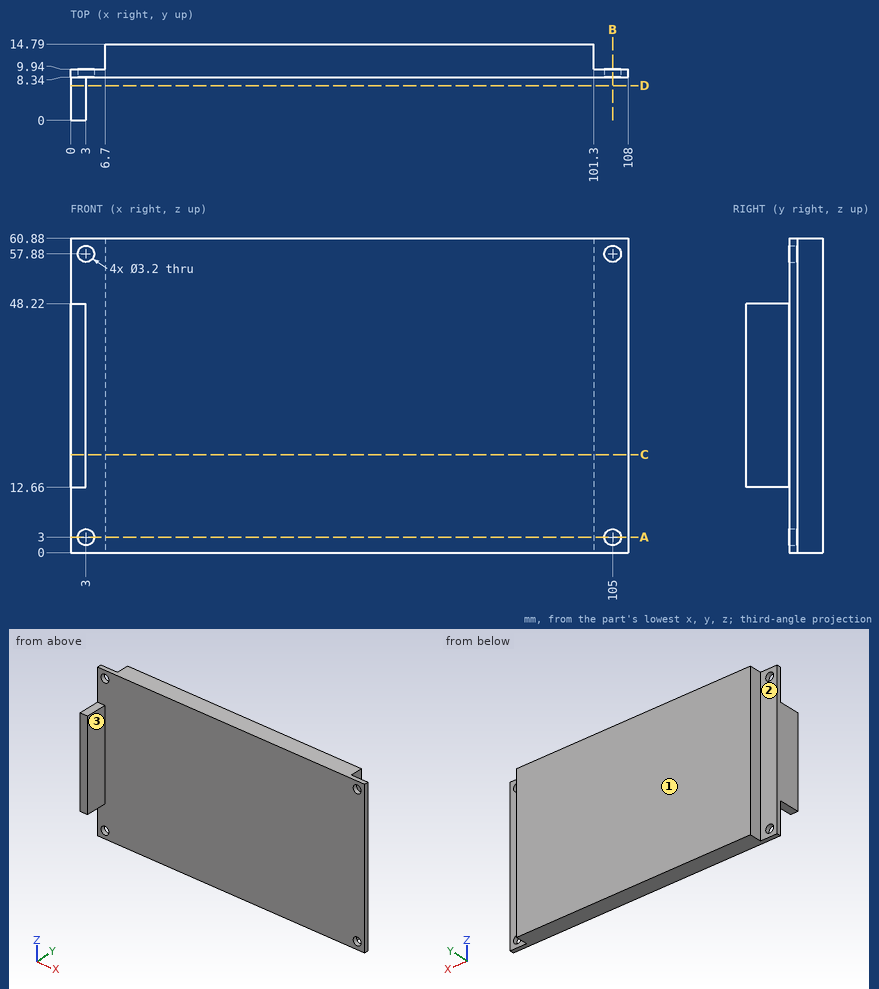
The figure shows three views and two pictorial views of one solid part (mm, origin at its lowest corner). Answer the questions. A direction names the side the tool comes from. Round coordinates to 2 decimals unless told otherwise and drop trailing zeros. Write each loop counter-clockwise with the first axis right and the second up, starting at its lowest first coordinate (ties: lowest second). Pieces come first, ordered by that corner, then holes. Notation, with made-up numbers: (-31, 5.5) -> (9, 5.5) arc R18 cw to (9, 13.5) -> close; hole circle Ø10 at (3, 42.5). An arc over 180 degrees is marked (long way). Write each question's results on one line, items separated by ' | '.
Q1. Section B-B, the plane x = 105 is taken. Write down the section's boundary in (y, z).
Data:
outline: (8.34, 0) -> (9.94, 0) -> (9.94, 1.4) -> (8.34, 1.4) -> close; (8.34, 4.6) -> (9.94, 4.6) -> (9.94, 56.28) -> (8.34, 56.28) -> close; (8.34, 59.48) -> (9.94, 59.48) -> (9.94, 60.88) -> (8.34, 60.88) -> close
Q2. Section C-C, the plane z = 19 is taken. Write down the section's boundary in (x, y).
Data:
outline: (0, 0) -> (3, 0) -> (3, 8.34) -> (108, 8.34) -> (108, 9.94) -> (101.3, 9.94) -> (101.3, 14.79) -> (6.7, 14.79) -> (6.7, 9.94) -> (0, 9.94) -> close
Q3. Flat-ended cylindrical pins translate along their axes: P1, Ø18.5, axis at x = 42, z = 28, coming from the -Y side; P2, Ø0.9, axis at x = 1.5, y = 2.5, coming from the -Z side; P3, Ø5.5, axis at y = 12, z = 19.5, coming from the -X side; P4, Ø3.5, axis at x = 104.5, z = 37, coming from the +Y side. Find the tip coordinate at first contact, or state that the pin passes through.
Data:
P1: y = 8.34 | P2: z = 12.66 | P3: x = 0 | P4: y = 9.94
Q4. Which of the six approach directions +Z, -Z, +X, -X, +Y, -Y give full straight-line access (tool end or side, diameter ignored) to the marked faces 1, 2 and 3?
Data:
face 1: +Z, -Z, +X, -X, +Y | face 2: +Z, -Z, -X, +Y | face 3: +Z, -Z, +X, -Y
Q5. Straight lines are drawn through the part: line 1 along X through (y, z) = (9.05, 3); line 2 along Z through (x, y) = (105, 8.75); line 3 along X through (y, z) = (5.25, 16.5). For each, find the intervals that lie inside material, in ascending order. Write a range as [from, to].
Data:
line 1: [0, 1.4], [4.6, 103.4], [106.6, 108] | line 2: [0, 1.4], [4.6, 56.28], [59.48, 60.88] | line 3: [0, 3]
Q6. Section A-A, the plane z = 3 is taken. Write down the section's boundary in (x, y).
Data:
outline: (0, 8.34) -> (1.4, 8.34) -> (1.4, 9.94) -> (0, 9.94) -> close; (4.6, 8.34) -> (103.4, 8.34) -> (103.4, 9.94) -> (101.3, 9.94) -> (101.3, 14.79) -> (6.7, 14.79) -> (6.7, 9.94) -> (4.6, 9.94) -> close; (106.6, 8.34) -> (108, 8.34) -> (108, 9.94) -> (106.6, 9.94) -> close
Q7. Section D-D, the plane y = 6.75 is taken. Write down the section's boundary in (x, z), then the cut area to 3 significant figures.
Data:
outline: (0, 12.66) -> (3, 12.66) -> (3, 48.22) -> (0, 48.22) -> close | area: 107 mm^2
